```python
from build123d import *

# Parameters (mm, degrees)
F0_R     = 5.15
F1_DEPTH = 35
F3_D     = 4.3
F4_R     = 3
F5_R     = 1.5


with BuildPart() as f1:
    # F0 (on Top) → F1 (new body)
    with BuildSketch(Plane.XY):
        with BuildLine():
            ThreePointArc((0, -7.15), (5.055813, -5.055813), (7.15, 0))
            ThreePointArc((7.15, 0), (5.055813, 5.055813), (0, 7.15))
            ThreePointArc((0, 7.15), (-7.15, 0), (0, -7.15))
        make_face()
        Circle(F0_R, mode=Mode.SUBTRACT)
        with BuildLine():
            Line((8, 0), (7.15, 0))
            ThreePointArc((7.15, 0), (5.055813, -5.055813), (0, -7.15))
            Line((0, -7.15), (6, -7.15))
            Line((6, -7.15), (6, -14))
            Line((6, -14), (8, -14))
            Line((8, -14), (8, 0))
        make_face()
        with BuildLine():
            ThreePointArc((0, 7.15), (5.055813, 5.055813), (7.15, 0))
            Line((7.15, 0), (8, 0))
            Line((8, 0), (8, 7.15))
            Line((8, 7.15), (0, 7.15))
        make_face()
    extrude(amount=F1_DEPTH)

    # F3 (through all)
    with Locations(Plane(origin=(6, 0, 0), x_dir=(0, -1, 0), z_dir=(-1, 0, 0))):
        with Locations((11.55, 8), (11.55, 27)):
            Hole(F3_D / 2)

    # F4
    f4_edges = [f1.edges().sort_by_distance(p)[0] for p in [
        (7, -14, 0),
        (7, -14, 35),
    ]]
    fillet(f4_edges, radius=F4_R)

    # F5
    f5_edges = [f1.edges().sort_by_distance(p)[0] for p in [
        (-5.15, 0, 0),
    ]]
    fillet(f5_edges, radius=F5_R)


solid = f1.part
```
Source: CAD feature listing. Evaluate the final solid. Frame: model axes, mm. A direction names the side the tool comes from. Round coordinates to 2 decimals unless told otherwise and drop trailing zeros. Loops run counter-clockwise (first coordinate to the right, second up) from the corner with the lowest first, then second, coordinate; pieces in that order, holes last.
1. Section query A-A on z = 8. Output: boundary loops of the cut face in (x, y), and give its area (3 significant figures).
2. Contact query for flat-ended pins moving along their axis: pin 1 (3 mm diameter, centred on x = 2, z = 11.5, fed in from -Y); pin 2 (7 mm diameter, centred on y = -11.55, z = 8, fed in from -X). Output: stop coordinate, or through.
3. Access query for faces 4 (the flat face through (5.4, 0.2, 35)), 5 (the flat face through (6, -11, 17)). Directions: +Z, -Z, +X, -X, +Y, -Y. A direction counts if a zero-diameter tool reaches every point of the face in a straight line with its end or side. Return the directions, or none.
4. Ray query, L1, parallel to Z at x = 6.55, y = -11.55; L2, parallel to X at y = -12, z = 5.5; L3, parallel to X at y = -0.25, z = 22.5. Return the intervals inside material, ascending.
5. Section query B-B on z = 12.5. Output: boundary loops of the cut face in (x, y), and give its area (3 significant figures).
6. Mould query, pull axis Z, two halves, no side actions, for faces 1 (the cylindrical face through (7.01, -13.1, 0.86)), 2 (the cylindrical face through (4.91, 1.55, 18.02)), 3 (the cylindrical face through (7.01, -11.83, 10.13)). Classes: released by +Z, released by -Z, zero draft, split by the parting line, or undercut.
7. Section query C-C on y = -11.55. Output: boundary loops of the cut face in (x, z), and give its area (3 significant figures).
Answers below:
1. outline: (0, -7.15) - (6, -7.15) - (6, -9.4) - (8, -9.4) - (8, 7.15) - (0, 7.15) arc R7.15 ccw to start; (6, -14) - (8, -14) - (8, -13.7) - (6, -13.7) - close; hole circle Ø10.3 at (0, 0)
1. area: 116 mm2
2. pin 1: stops at y = -7.15
2. pin 2: stops at x = 6
3. face 4: +Z, +X, -X, +Y, -Y
3. face 5: +Z, -Z, -X, -Y
4. L1: z = 0.05 to 5.85, 10.15 to 24.85, 29.15 to 34.95
4. L2: x = 6 to 8
4. L3: x = -7.15 to -5.14, 5.14 to 8
5. outline: (0, -7.15) - (6, -7.15) - (6, -14) - (8, -14) - (8, 7.15) - (0, 7.15) arc R7.15 ccw to start; hole circle Ø10.3 at (0, 0)
5. area: 125 mm2
6. face 1: released by -Z
6. face 2: zero draft
6. face 3: undercut
7. outline: (6, 0.05) - (8, 0.05) - (8, 5.85) - (6, 5.85) - close; (6, 10.15) - (8, 10.15) - (8, 24.85) - (6, 24.85) - close; (6, 29.15) - (8, 29.15) - (8, 34.95) - (6, 34.95) - close
7. area: 52.6 mm2
